from build123d import *

# Parameters (mm, degrees)
BASE_FLANGE1_DEPTH            = 3.175
EDGE_FLANGE1_STRIP_W          = 19.05
EDGE_FLANGE1_STRIP_H          = 3.175
EDGE_FLANGE1_STRIP_CUT_DEPTH  = 37.325997284
EDGE_FLANGE1_RELIEF_W         = 20.6375
EDGE_FLANGE1_RELIEF_H         = 1.5875
EDGE_FLANGE1_RELIEF_CUT_DEPTH = 3.175
EDGE_FLANGE1_DEPTH            = 37.325997284
SKETCH15_R                    = 2.65
CUT_EXTRUDE2_DEPTH            = 10
SKETCH19_R                    = 3.15
CUT_EXTRUDE4_DEPTH            = 10


# Sheet-metal steps are written as plain solids
with BuildPart() as part:
    # Sketch3 → Base-Flange1 (new body)
    with BuildSketch(Plane(origin=(0, 0, 0), x_dir=(0, 0, -1), z_dir=(1, 0, 0))):
        with BuildLine():
            Line((83.106142408, 32.105064535), (45.780209905, 32.174606262))
            Line((45.780209905, 32.174606262), (45.780209905, 43.136168925))
            ThreePointArc((45.780209905, 43.136168925), (46.495831721, 45.713784796), (48.437851335, 47.553561406))
            Line((48.437851335, 47.553561406), (83.169236275, 65.970162941))
            Line((83.169236275, 65.970162941), (83.106142408, 32.105064535))
        make_face()
    extrude(amount=-BASE_FLANGE1_DEPTH)

    # Edge-Flange1 strip (across the edge) → Edge-Flange1 strip cut (cut)
    with BuildSketch(Plane(origin=(-3.175, 32.105064535, -83.106142408), x_dir=(-3.4914813388431334e-15, 0.999998264444559, -0.001863090945206598), z_dir=(0, 0.001863090945206598, 0.999998264444559))):
        with Locations((-3.175, -1.5875)):
            Rectangle(EDGE_FLANGE1_STRIP_W, EDGE_FLANGE1_STRIP_H)
    extrude(amount=EDGE_FLANGE1_STRIP_CUT_DEPTH, mode=Mode.SUBTRACT)

    # Edge-Flange1 relief (on the sheet) → Edge-Flange1 relief cut (cut)
    with BuildSketch(Plane(origin=(-3.175, 38.455053514, -83.117973035), x_dir=(-6.982962677686267e-15, 0.999998264444559, -0.001863090945206598), z_dir=(-1, 0, 0))):
        with Locations((-8.73125, -38.119747284)):
            Rectangle(EDGE_FLANGE1_RELIEF_W, EDGE_FLANGE1_RELIEF_H)
    extrude(amount=-EDGE_FLANGE1_RELIEF_CUT_DEPTH, mode=Mode.SUBTRACT)

    # Edge-Flange1 section (across the edge) → Edge-Flange1 (add)
    with BuildSketch(Plane(origin=(-3.175, 32.105064535, -83.106142408), x_dir=(-3.4914813388431334e-15, 0.999998264444559, -0.001863090945206598), z_dir=(0, 0.001863090945206598, 0.999998264444559))):
        with BuildLine():
            Line((0, 3.175), (0, 15))
            Line((0, 15), (3.175, 15))
            Line((3.175, 15), (3.175, 3.175))
            ThreePointArc((3.175, 3.175), (4.10493597, 0.92993597), (6.35, 0))
            Line((6.35, 0), (6.35, -3.175))
            ThreePointArc((6.35, -3.175), (1.859871939, -1.315128061), (0, 3.175))
        make_face()
    extrude(amount=EDGE_FLANGE1_DEPTH)

    # Sketch15 → Cut-Extrude2 (cut)
    with BuildSketch(Plane(origin=(0, 35.434781617, -0.066018335), x_dir=(1, 0, 0), z_dir=(-3.23986857388729e-15, 0.999998264444559, -0.0018630909452065992))):
        with Locations(Location((-12.2625, 64.389781839, 0), (0, 0, 270))):
            Circle(SKETCH15_R)
    extrude(amount=-CUT_EXTRUDE2_DEPTH, mode=Mode.SUBTRACT)

    # Sketch19 → Cut-Extrude4 (cut)
    with BuildSketch(Plane.ZY.offset(3.175)):
        with Locations((-74.30640548, 51.024595242)):
            Circle(SKETCH19_R)
        with Locations((-54.306440614, 43.524595242)):
            Circle(SKETCH19_R)
    extrude(amount=-CUT_EXTRUDE4_DEPTH, mode=Mode.SUBTRACT)


solid = part.part
For this review, take the finished solid that the model builds, in its own axes (mm). A direction names the side the tool comes from. Coordinates: 2 decimals unless noted, no trailing zeros. Loops run counter-clockwise (first coordinate to the right, second up) from the corner with the lowest first, then second, coordinate; pieces in that order, holes last. Notation, with made-up numbers: (65, 26) - (118, 26) arc R14 ccw to (118, 35) - close; hole circle Ø10 at (3, 5.25). An arc over 180 degrees is marked (long way). Use a Markdown table: item, result. Add a question column.
Item 1: Insertion check: pin 1 Ø5.5 at (y, z) = (43.52, -54.31) entering from +X; pin 2 Ø5 at (x, z) = (-12, -64.5) entering from -Y; pin 3 Ø1.5 at (y, z) = (52, -69) entering from -X (3 decimals); pin 4 Ø2 at (x, z) = (-3, -60.5) entering from +Y. Each pin has a flat end and moves straight along its axis. Give the tip position at first contact, or say it passes through.
Item 2: We need section D-D (y = 63.5). Give the boundary of the cut face in (x, z) (3 decimals), and give its area (3 significant figures).
Item 3: For line 1 (X direction, y = 41.5, z = -49) (3 decimals); line 2 (Y direction, x = -15.75, z = -67); line 3 (Z direction, x = -3, y = 46), list the stretches that pass through material, from the lowest coordinate up.
Item 4: We need section B-B (x = -2.5). Give the boundary of the cut face in (y, z) (3 decimals), and give its area (3 significant figures).
Item 5: We need section A-A (x = -11.5). Give the boundary of the cut face in (y, z), and give its area (3 significant figures).
Item 6: Tool access review of faces 4 (the face through (-4.13, 36.22, -64.71)), 5 (the face through (-1.81, 34.05, -64.71)), 6 (the face through (-1.565, 56.633, -65.56)): name each direction out of +Z, -Z, +X, -X, +Y, -Y from which nothing blocks a thin tool from reaching the whole face with its end or side.
Item 7: We need section C-C (y = 55). Give the boundary of the cut face in (x, z) (3 decimals).
Item 8: Mouldability with a two-part tool opening along Y and no side actions: class faces 1 (the face through (-1.565, 45.681, -46.476)), 2 (the face through (-3.175, 49, -69)), 3 (the face through (-1.61, 49.818, -71.397)) as pulls with the +Y half, pulls with the -Y half, needs draft (parallel to the pull), parting line crosses it, or undercut.
Results list:
| question | item | result |
|---|---|---|
| 1 | pin 1 | passes through |
| 1 | pin 2 | stops at y = 32.14 |
| 1 | pin 3 | stops at x = -3.175 |
| 1 | pin 4 | stops at y = 54.48 |
| 2 | outline | (-3.175, -83.165) - (0, -83.165) - (0, -78.511) - (-3.175, -78.511) - close |
| 2 | area | 14.8 mm^2 |
| 3 | line 1 | x = -3.175 to 0 |
| 3 | line 2 | y = 32.14 to 35.31 |
| 3 | line 3 | z = -83.13 to -56.25, -52.36 to -46.68 |
| 4 | outline | (33.405, -83.109) - (65.97, -83.169) - (47.554, -48.438) arc R5 ccw to (43.136, -45.78) - (40.112, -45.78) - (40.112, -45.795) - (33.475, -45.783) - close; hole circle Ø6.3 at (43.525, -54.306); hole circle Ø6.3 at (51.025, -74.306) |
| 4 | area | 781 mm^2 |
| 5 | outline | (32.11, -83.11) - (35.28, -83.11) - (35.31, -66.99) - (32.14, -66.99) - close; (32.14, -61.91) - (35.32, -61.92) - (35.35, -45.79) - (32.17, -45.78) - close |
| 5 | area | 102 mm^2 |
| 6 | face 4 | -Z, -X, +Y |
| 6 | face 5 | +Z, +X, -Y |
| 6 | face 6 | +Z, +X, -X, +Y |
| 7 | outline | (-3.175, -83.149) - (0, -83.149) - (0, -62.481) - (-3.175, -62.481) - close |
| 8 | face 1 | pulls with the +Y half |
| 8 | face 2 | needs draft |
| 8 | face 3 | undercut |
